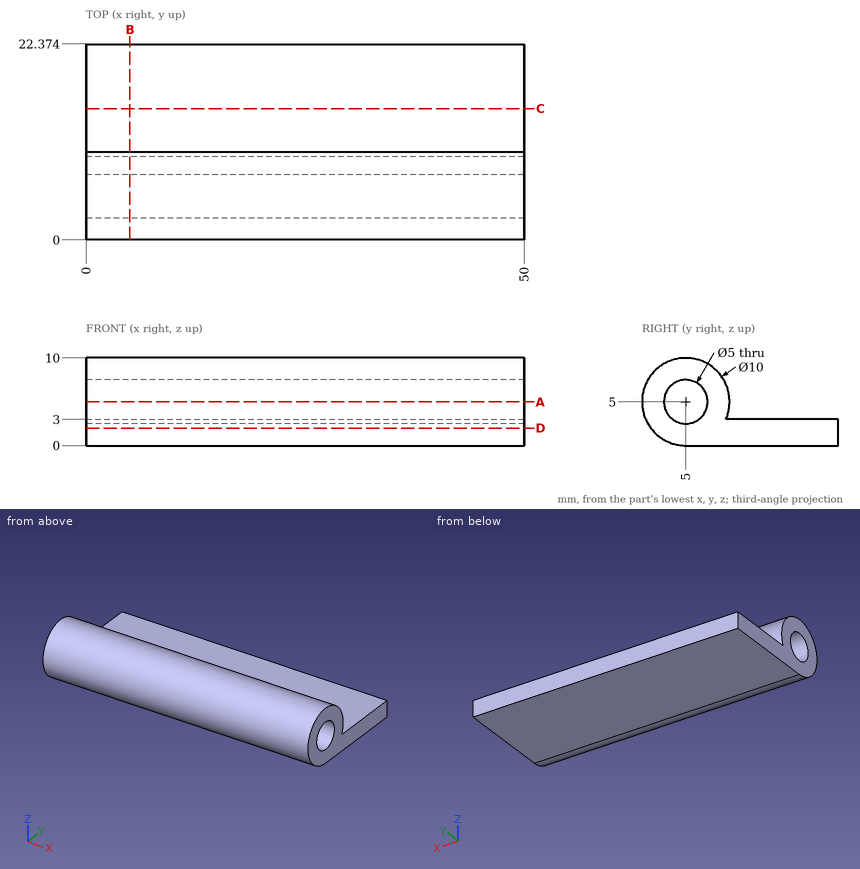
Can you work these out from the drawing? Everything is in mm from the part's minimum corner. Round coordinates to 2 decimals unless told otherwise and drop trailing zeros. Loops run counter-clockwise (first coordinate to the right, second up) from the corner with the lowest first, then second, coordinate; pieces in that order, holes last.
1. If I drill on line 1 along Z through (x, y) = (11, 5); line 2 along Y through (x, z) = (13.5, 5.75) (1 decimal); line 3 along Z through (x, y) = (38, 2.75) (1 decimal), over which ranges is the centre line in solid material (lowest first)?
Answer list:
line 1: z = 0 to 2.5, 7.5 to 10
line 2: y = 0.1 to 2.6, 7.4 to 9.9
line 3: z = 0.5 to 3.9, 6.1 to 9.5
2. For P1, Ø6, axis at x = 11, y = 15.5, coming from the +Z side; P2, Ø2, axis at x = 34, z = 2, coming from the -Y side; P3, Ø1, axis at y = 11, z = 6.5, coming from the -X side; P4, Ø12, axis at x = 19.5, y = 14.5, coming from the +Z side, each with a flat end and sliding along its axis, tell me the tip position at first contact or that it passes through.
Answer list:
P1: stops at z = 3
P2: stops at y = 0.42
P3: passes through
P4: stops at z = 8.57
3. If we section it at A-A on z = 5: Write out the boundary of the cut face in (x, y), plus the area to 3 significant figures.
Answer list:
outline: (0, 0) - (50, 0) - (50, 2.5) - (0, 2.5) - close; (0, 7.5) - (50, 7.5) - (50, 10) - (0, 10) - close
area: 250 mm2
4. If we section it at B-B on x = 5: Write out the boundary of the cut face in (y, z).
Answer list:
outline: (5, 0) - (22.37, 0) - (22.37, 3) - (9.58, 3) arc R5 ccw (long way) to start; hole circle Ø5 at (5, 5)
5. If we section it at D-D on z = 2: Write out the boundary of the cut face in (x, y).
Answer list:
outline: (0, 1) - (50, 1) - (50, 22.37) - (0, 22.37) - close
6. If we section it at C-C on y = 15: Write out the boundary of the cut face in (x, z).
Answer list:
outline: (0, 0) - (50, 0) - (50, 3) - (0, 3) - close
